Read the model definition and answer for the solid it produces. Units are mm, in the model's axes. A direction names the side the tool comes from. Coordinates: 2 decimals unless noted, no trailing zeros. Write each loop counter-clockwise with the first axis right and the second up, starting at its lowest first coordinate (ties: lowest second). Pieces come first, ordered by that corner, then holes. Notation, with made-up numbers: (51.5, -9.75) -> (72.5, -9.75) arc R17 ccw to (72.5, -3.75) -> close; hole circle Ø4 at (-40, 54). An arc over 180 degrees is marked (long way). Answer in a Markdown table with one row per item. Add a question column.
Item 1: Section A-A on x = 45 is taken. Write down the section's boundary in (y, z).
Item 2: Which of the six approach directions +Z, -Z, +X, -X, +Y, -Y give full straight-line access (tool end or side, diameter ignored) to faces 5 (the face through (-8, -73, 5)), 6 (the face through (-77.9, 68, 2.5))?
Item 3: Given pin 1 Ø16 at (x, y) = (-45, 80) entering from -Z, flat-ended and moving along its own axis, determine where the tip first touches the part or whether it passes through.
Item 4: Straight lines are drawn through the part: line 1 (Y direction, x = 90, z = 1.1); line 2 (X direction, y = 52.5, z = 3.5); line 3 (Y direction, x = 59.5, z = 2.1). For each, find the intervals that lie inside material, in ascending order. Write a range as from..to.
Item 5: For a pull along X with two mould halves and no side action, classify faces 1 (the face through (77.9, -68, 2.5)), 2 (the face through (97.15, 86.99, 2.46)), 3 (the face through (1, 90, 2)), 4 (the face through (-97.15, -86.99, 2.46)) as +X half, -X half, draft (parallel to the pull), parting line (faces both ways), or undercut.
Item 6: Section D-D on x = -65 is taken. Write down the section's boundary in (y, z), then the cut area to 3 significant figures.
Item 7: Section C-C on z = 1.6 is taken. Count the separate pieces of the cut face and the enclosed holes in it, then the cut area to 3 significant figures.
Item 8: Section B-B on y = -31 is taken. Write down the section's boundary in (x, z), then the cut area to 3 significant figures.
```python
from build123d import *

# Parameters (mm, degrees)
SKETCH_1_R      = 5
EXTRUDE_1_DEPTH = 5


with BuildPart() as part:
    # 草图1 → 凸台-拉伸1 (new body)
    with BuildSketch(Plane.XY):
        with BuildLine():
            Line((-90, -90), (90, -90))
            ThreePointArc((90, -90), (97.071067812, -87.071067812), (100, -80))
            Line((100, -80), (100, 80))
            ThreePointArc((100, 80), (97.071067812, 87.071067812), (90, 90))
            Line((90, 90), (-90, 90))
            ThreePointArc((-90, 90), (-97.071067812, 87.071067812), (-100, 80))
            Line((-100, 80), (-100, -80))
            ThreePointArc((-100, -80), (-97.071067812, -87.071067812), (-90, -90))
        make_face()
        with Locations((90, -80)):
            Circle(SKETCH_1_R, mode=Mode.SUBTRACT)
        with Locations((90, 80)):
            Circle(SKETCH_1_R, mode=Mode.SUBTRACT)
        with Locations((-90, 80)):
            Circle(SKETCH_1_R, mode=Mode.SUBTRACT)
        with Locations((-90, -80)):
            Circle(SKETCH_1_R, mode=Mode.SUBTRACT)
        with Locations((90, 0)):
            Circle(SKETCH_1_R, mode=Mode.SUBTRACT)
        with Locations((90, -40)):
            Circle(SKETCH_1_R, mode=Mode.SUBTRACT)
        with Locations((90, 40)):
            Circle(SKETCH_1_R, mode=Mode.SUBTRACT)
        with Locations(Location((-90, -40, 0), (0, 0, 180))):
            Circle(SKETCH_1_R, mode=Mode.SUBTRACT)
        with Locations(Location((-90, 0, 0), (0, 0, 180))):
            Circle(SKETCH_1_R, mode=Mode.SUBTRACT)
        with Locations(Location((-90, 40, 0), (0, 0, 180))):
            Circle(SKETCH_1_R, mode=Mode.SUBTRACT)
        with Locations((0, 80)):
            Circle(SKETCH_1_R, mode=Mode.SUBTRACT)
        with Locations((-45, 80)):
            Circle(SKETCH_1_R, mode=Mode.SUBTRACT)
        with Locations((45, 80)):
            Circle(SKETCH_1_R, mode=Mode.SUBTRACT)
        with Locations((0, -80)):
            Circle(SKETCH_1_R, mode=Mode.SUBTRACT)
        with Locations((-45, -80)):
            Circle(SKETCH_1_R, mode=Mode.SUBTRACT)
        with Locations((45, -80)):
            Circle(SKETCH_1_R, mode=Mode.SUBTRACT)
        with BuildLine():
            Line((-73, -70), (73, -70))
            ThreePointArc((73, -70), (77.949747468, -67.949747468), (80, -63))
            Line((80, -63), (80, 63))
            ThreePointArc((80, 63), (77.949747468, 67.949747468), (73, 70))
            Line((73, 70), (-73, 70))
            ThreePointArc((-73, 70), (-77.949747468, 67.949747468), (-80, 63))
            Line((-80, 63), (-80, -63))
            ThreePointArc((-80, -63), (-77.949747468, -67.949747468), (-73, -70))
        make_face(mode=Mode.SUBTRACT)
    extrude(amount=EXTRUDE_1_DEPTH)


solid = part.part
```
Results below:
| question | item | result |
|---|---|---|
| 1 | outline | (-90, 0) -> (-85, 0) -> (-85, 5) -> (-90, 5) -> close; (-75, 0) -> (-70, 0) -> (-70, 5) -> (-75, 5) -> close; (70, 0) -> (75, 0) -> (75, 5) -> (70, 5) -> close; (85, 0) -> (90, 0) -> (90, 5) -> (85, 5) -> close |
| 2 | face 5 | +Z, +X, -X, +Y, -Y |
| 2 | face 6 | +Z, -Z |
| 3 | pin 1 | stops at z = 0 |
| 4 | line 1 | y = -90..-85, -75..-45, -35..-5, 5..35, 45..75, 85..90 |
| 4 | line 2 | x = -100..-80, 80..100 |
| 4 | line 3 | y = -90..-70, 70..90 |
| 5 | face 1 | undercut |
| 5 | face 2 | +X half |
| 5 | face 3 | draft |
| 5 | face 4 | -X half |
| 6 | outline | (-90, 0) -> (-70, 0) -> (-70, 5) -> (-90, 5) -> close; (70, 0) -> (90, 0) -> (90, 5) -> (70, 5) -> close |
| 6 | area | 200 mm2 |
| 7 | separate pieces | 1 |
| 7 | enclosed holes | 17 |
| 7 | area | 12,300 mm2 |
| 8 | outline | (-100, 0) -> (-80, 0) -> (-80, 5) -> (-100, 5) -> close; (80, 0) -> (100, 0) -> (100, 5) -> (80, 5) -> close |
| 8 | area | 200 mm2 |
